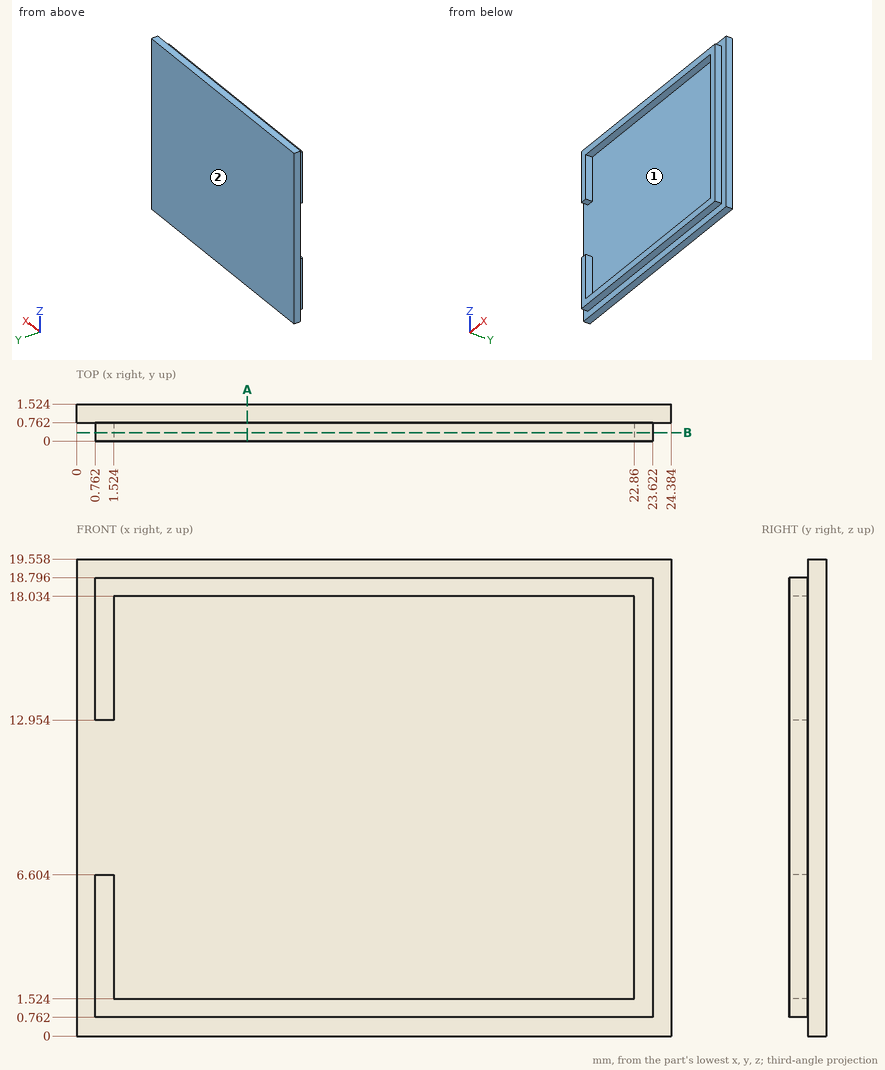
Could you check a few things on this drawing? It's one solid part, dimensions in mm from its lowest x, y, z. Give positions to 0.01 mm unless a question says otherwise; leave off trailing zeros. Loops run counter-clockwise (first coordinate to the right, second up) from the corner with the lowest first, then second, coordinate; pieces in that order, holes last. Notation, with made-up numbers: M 14,-1.75 L 54,-1.75 A8 cw 54,13.25 Z; hole C 79,3 d3. An arc over 180 degrees is marked long. Answer as a JSON object with one key per item and string values.
Q1. If we mould it in two halves opening along X, with no side actions, what happens to the marked faces 1 and 2? For each: pulls with the +X half, pulls with the -X half, needs draft (parallel to the pull), parting line crosses it, or undercut.
Values found:
{"face 1": "undercut", "face 2": "needs draft"}
Q2. Suppose I cut it at A-A, the plane x = 7. List the corners of the cut face in (y, z) for me, plus the area to 3 significant figures.
Values found:
{"outline": "M 0,0.76 L 0.76,0.76 L 0.76,0 L 1.52,0 L 1.52,19.56 L 0.76,19.56 L 0.76,18.8 L 0,18.8 L 0,18.03 L 0.76,18.03 L 0.76,1.52 L 0,1.52 Z", "area": "16.1 mm²"}
Q3. Suppose I cut it at B-B, the plane y = 0.35. List the corners of the cut face in (x, z) for me.
Values found:
{"outline": "M 0.76,0.76 L 23.62,0.76 L 23.62,18.8 L 0.76,18.8 L 0.76,12.95 L 1.52,12.95 L 1.52,18.03 L 22.86,18.03 L 22.86,1.52 L 1.52,1.52 L 1.52,6.6 L 0.76,6.6 Z"}
Q4. For P1, Ø2, axis at x = 6, z = 16.5, coming from the -Y side; P2, Ø0.8, axis at y = 0, z = 5, coming from the +X side, each with a flat end and sliding along its axis, tell me the tip position at first contact or that it passes through.
Values found:
{"P1": "stops at y = 0.76", "P2": "stops at x = 23.62"}
Q5. If I drill on probe 1 along Z at (x, y) = (20.5, 0.5); probe 2 along X at (y, z) = (0.1, 14.5); probe 3 along X at (y, z) = (0.15, 10), over which ranges is the centre line in solid material (lowest first)? Write a range as [from, to].
Values found:
{"probe 1": "z = [0.76, 1.52], [18.03, 18.8]", "probe 2": "x = [0.76, 1.52], [22.86, 23.62]", "probe 3": "x = [22.86, 23.62]"}
